from build123d import *

# Parameters (mm, degrees)
IZIM2_W                     = 88.39
IZIM2_H                     = 59.7
Y_KSEKLIK_EKSTR_ZYON1_DEPTH = 4
Y_KSEKLIK_EKSTR_ZYON2_DEPTH = 7
Y_KSEKLIK_EKSTR_ZYON3_DEPTH = 4
RADYUS2_R                   = 4
IZIM6_R                     = 2.025
KES_EKSTR_ZYON1_DEPTH       = 4
RADYUS2_OF_AYNALAMA1_R      = 4
IZIM10_W                    = 5.1
IZIM10_H                    = 2
KES_EKSTR_ZYON2_DEPTH       = 88.39


with BuildPart() as part:
    # Çizim2 → Yükseklik-Ekstrüzyon1 (new body)
    with BuildSketch(Plane(origin=(0, 0, 0), x_dir=(1, 0, 0), z_dir=(0, 1, 0))):
        with Locations((5.778877035, -29.85)):
            Rectangle(IZIM2_W, IZIM2_H)
    extrude(amount=Y_KSEKLIK_EKSTR_ZYON1_DEPTH)

    # Çizim3 → Yükseklik-Ekstrüzyon2 (add)
    with BuildSketch(Plane(origin=(0, 4, 0), x_dir=(1, 0, 0), z_dir=(0, 1, 0))):
        with BuildLine():
            ThreePointArc((-38.416122965, -39.288399656), (-21.474324276, -29.85), (-38.416122965, -20.411600344))
            Line((-38.416122965, -20.411600344), (-38.416122965, -24.238994023))
            ThreePointArc((-38.416122965, -24.238994023), (-24.474324276, -29.85), (-38.416122965, -35.461005977))
            Line((-38.416122965, -35.461005977), (-38.416122965, -39.288399656))
        make_face()
    extrude(amount=Y_KSEKLIK_EKSTR_ZYON2_DEPTH)

    # Çizim5 → Yükseklik-Ekstrüzyon3 (add)
    with BuildSketch(Plane(origin=(19.973877035, 0, 0), x_dir=(0, 0, -1), z_dir=(1, 0, 0))):
        Polygon((-32.003216554, 4), (-27.696783446, 4), (-25.626729832, 4), (-25.626729832, 54), (-34.073270168, 54), (-34.073270168, 4), align=None)
    y_kseklik_ekstr_zyon3 = extrude(amount=Y_KSEKLIK_EKSTR_ZYON3_DEPTH)

    # Radyus2
    radyus2_edges = [part.edges().sort_by_distance(p)[0] for p in [
        (21.973877035, 54, 25.626729832),
        (21.973877035, 54, 34.073270168),
    ]]
    fillet(radyus2_edges, radius=RADYUS2_R)

    # Çizim6 → Kes-Ekstrüzyon1 (cut)
    with BuildSketch(Plane(origin=(23.973877035, 0, 0), x_dir=(0, 0, -1), z_dir=(1, 0, 0))):
        with Locations((-29.85, 50)):
            Circle(IZIM6_R)
    kes_ekstr_zyon1 = extrude(amount=-KES_EKSTR_ZYON1_DEPTH, mode=Mode.SUBTRACT)

    # Aynalama1: Yükseklik-Ekstrüzyon3, Kes-Ekstrüzyon1 across plane
    add(y_kseklik_ekstr_zyon3.mirror(Plane(origin=(4.973877035, 0, 0), x_dir=(0, 0, 1), z_dir=(1, 0, 0))))
    add(kes_ekstr_zyon1.mirror(Plane(origin=(4.973877035, 0, 0), x_dir=(0, 0, 1), z_dir=(1, 0, 0))), mode=Mode.SUBTRACT)

    # Radyus2 of Aynalama1
    radyus2_of_aynalama1_edges = [part.edges().sort_by_distance(p)[0] for p in [
        (-12.026122965, 54, 25.626729832),
        (-12.026122965, 54, 34.073270168),
    ]]
    fillet(radyus2_of_aynalama1_edges, radius=RADYUS2_OF_AYNALAMA1_R)

    # Çizim10 → Kes-Ekstrüzyon2 (cut)
    with BuildSketch(Plane.ZY.offset(38.416122965)):
        with Locations((2.55, 1)):
            Rectangle(IZIM10_W, IZIM10_H)
        with Locations((57.15, 1)):
            Rectangle(IZIM10_W, IZIM10_H)
    extrude(amount=-KES_EKSTR_ZYON2_DEPTH, mode=Mode.SUBTRACT)


solid = part.part
Input: part model. Units: mm. Frame: model coordinates. A direction names the side the tool comes from. Coordinates: 2 decimals unless noted, no trailing zeros. Order: outer loops, then holes, each group sorted by start corner. A loop starts at its lowest first (then second) coordinate and runs counter-clockwise, first axis right, second up.
1. Ray query, line 1 along X through (y, z) = (20, 31.5); line 2 along X through (y, z) = (5, 29); line 3 along Y through (x, z) = (22, 29). Return the intervals inside material, ascending.
Checked values:
line 1: x = -14.03 to -10.03, 19.97 to 23.97
line 2: x = -24.52 to -21.51, -14.03 to -10.03, 19.97 to 23.97
line 3: y = 0 to 48.16, 51.84 to 53.95
2. Cut plane A-A, the plane y = 35. Return loops of the section in (x, z), plus the area to 3 significant figures.
Checked values:
outline: (-14.03, 25.63) - (-10.03, 25.63) - (-10.03, 34.07) - (-14.03, 34.07) - close; (19.97, 25.63) - (23.97, 25.63) - (23.97, 34.07) - (19.97, 34.07) - close
area: 67.6 mm2
3. Cut plane B-B, the plane x = 27. Return loops of the section in (y, z), plus the area to 3 significant figures.
Checked values:
outline: (0, 5.1) - (2, 5.1) - (2, 0) - (4, 0) - (4, 59.7) - (2, 59.7) - (2, 54.6) - (0, 54.6) - close
area: 218 mm2
4. Cut plane D-D, the plane y = 7. Return loops of the section in (x, z), plus the area to 3 significant figures.
Checked values:
outline: (-38.42, 20.41) arc R11.1 ccw (long way) to (-38.42, 39.29) - (-38.42, 35.46) arc R8.1 cw (long way) to (-38.42, 24.24) - close; (-14.03, 25.63) - (-10.03, 25.63) - (-10.03, 34.07) - (-14.03, 34.07) - close; (19.97, 25.63) - (23.97, 25.63) - (23.97, 34.07) - (19.97, 34.07) - close
area: 196 mm2
5. Access query for faces 1 (the cylindrical face through (-24.48, 7.45, 29.58)), 2 (the flat face through (5, 2, 57)), 3 (the flat face through (23.974, 29, 30)), 4 (the flat face through (5, 2, 3)), 5 (the flat face through (-24, 11, 30)). Directions: +Z, -Z, +X, -X, +Y, -Y. A direction counts if a zero-diameter tool reaches every point of the face in a straight line with its end or side. Return the directions, or none.
Checked values:
face 1: +Y
face 2: +Z, +X, -X, -Y
face 3: +Z, -Z, +X, +Y
face 4: -Z, +X, -X, -Y
face 5: +Z, -Z, -X, +Y
6. Draft query along Z for faces 6 (the cylindrical face through (22, 50.61, 27.92)), 7 (the flat face through (5, 1, 54.6)), 8 (the cylindrical face through (-12.05, 52.8, 26.77)). Return one class per face: +Z half, -Z half, draft (parallel to the pull), parting line (faces both ways), or undercut.
Checked values:
face 6: undercut
face 7: +Z half
face 8: -Z half
7. Contact query for flat-ended pins moving along their axis: P1, Ø3, axis at x = -13, y = 37.5, coming from the +Z side; P2, Ø3, axis at x = -11, y = 37.5, coming from the -Z side; P3, Ø4, axis at y = 39.5, z = 30.5, coming from the +X side. Output: stop coordinate, or through.
Checked values:
P1: stops at z = 34.07
P2: stops at z = 25.63
P3: stops at x = 23.97
8. Cut plane C-C, the plane z = 52. Return loops of the section in (x, y), plus the area to 3 significant figures.
Checked values:
outline: (-38.42, 0) - (49.97, 0) - (49.97, 4) - (-38.42, 4) - close
area: 354 mm2
